from build123d import *

# Parameters (mm, degrees)
BOSS_EXTRUDE1_DEPTH = 6.35
SKETCH2_W           = 20
SKETCH2_H           = 6.55
CUT_EXTRUDE1_DEPTH  = 172.94569637
SKETCH4_W           = 6.55
SKETCH4_H           = 15
SKETCH4_W_2         = 6.35
CUT_EXTRUDE2_DEPTH  = 172.94569637
FILLET1_R           = 2


with BuildPart() as part:
    # Sketch1 → Boss-Extrude1 (new body)
    with BuildSketch(Plane(origin=(0, 0, 0), x_dir=(1, 0, 0), z_dir=(0, 1, 0))):
        Polygon((-170, 0), (-170, 20), (0, 20), (7, 20), (7, -25), (0, -25), (-170, -25), align=None)
    extrude(amount=BOSS_EXTRUDE1_DEPTH)

    # Sketch2 → Cut-Extrude1 (cut, through all)
    with BuildSketch(Plane(origin=(0, 6.35, 0), x_dir=(1, 0, 0), z_dir=(0, 1, 0))):
        with Locations((-110, -16.725)):
            Rectangle(SKETCH2_W, SKETCH2_H)
        with Locations((-155, -16.725)):
            Rectangle(SKETCH2_W, SKETCH2_H)
        with Locations((-65, -16.725)):
            Rectangle(SKETCH2_W, SKETCH2_H)
        with Locations((-20, -16.725)):
            Rectangle(SKETCH2_W, SKETCH2_H)
        with Locations((-110, -3.275)):
            Rectangle(SKETCH2_W, SKETCH2_H)
        with Locations((-155, -3.275)):
            Rectangle(SKETCH2_W, SKETCH2_H)
        with Locations((-65, -3.275)):
            Rectangle(SKETCH2_W, SKETCH2_H)
        with Locations((-20, -3.275)):
            Rectangle(SKETCH2_W, SKETCH2_H)
    extrude(amount=-CUT_EXTRUDE1_DEPTH, mode=Mode.SUBTRACT)

    # Sketch4 → Cut-Extrude2 (cut, through all)
    with BuildSketch(Plane(origin=(0, 6.35, 0), x_dir=(1, 0, 0), z_dir=(0, 1, 0))):
        with Locations((0, -12.5)):
            Rectangle(SKETCH4_W, SKETCH4_H)
        with Locations((0, 7.5)):
            Rectangle(SKETCH4_W_2, SKETCH4_H)
    extrude(amount=-CUT_EXTRUDE2_DEPTH, mode=Mode.SUBTRACT)

    # Fillet1
    fillet1_edges = [part.edges().sort_by_distance(p)[0] for p in [
        (7, 3.175, -20),
        (7, 3.175, 25),
        (-170, 3.175, 25),
        (-170, 3.175, -20),
    ]]
    fillet(fillet1_edges, radius=FILLET1_R)


solid = part.part
Could you check a few things on this model? Use its own coordinates, in mm. Coordinates: 2 decimals unless noted, no trailing zeros. Order: outer loops, then holes, each group sorted by start corner. A loop starts at its lowest first (then second) coordinate and runs counter-clockwise, first axis right, second up. Notation, with made-up numbers: (75.5, 16.25) -> (118.5, 16.25) arc R22 ccw to (118.5, 43.25) -> close; hole circle Ø10 at (87.25, 12.5). An arc over 180 degrees is marked (long way). One line per item, written item: value. Start each with the question number.
1) We'd pull the mould along X, two halves only. Please class faces 1 (the flat face through (0, 3, 0)), 2 (the flat face through (7, 3, 2)), 3 (the flat face through (-10, 3, 17)): +X half, -X half, draft (parallel to the pull), parting line (faces both ways), or undercut.
2) Imagine slicing it at A-A on x = -109. List the corners of the cut face in (y, z) for me, plus the area to 3 significant figures.
3) Imagine slicing it at C-C on y = 2. Count the separate pieces of the cut face and the enclosed holes in it, plus the area to 3 significant figures.
4) If I drill on L1, parallel to Z at x = -118, y = 2.5; L2, parallel to X at y = 5.25, z = 3.5; L3, parallel to X at y = 3, z = 16.5 (3 decimals), over which ranges is the centre line in solid material (lowest first)? Write a range as [from, to].
5) Imagine slicing it at B-B on z = -2. List the corners of the cut face in (x, y) for me (3 decimals), plus the area to 3 significant figures.
6) I'm going to push a flat-ended pin straight in: pin 1 (8 mm diameter, centred on x = -63, z = -8, fed in from -Y). Where does the tip first touch, or does it pass through?
Answer list:
1. face 1: undercut
1. face 2: +X half
1. face 3: undercut
2. outline: (0, -20) -> (6.35, -20) -> (6.35, 0) -> (0, 0) -> close; (0, 6.55) -> (6.35, 6.55) -> (6.35, 13.45) -> (0, 13.45) -> close; (0, 20) -> (6.35, 20) -> (6.35, 25) -> (0, 25) -> close
2. area: 203 mm2
3. separate pieces: 1
3. enclosed holes: 10
3. area: 6,720 mm2
4. L1: z = [-20, 0], [6.55, 13.45], [20, 25]
4. L2: x = [-170, -165], [-145, -120], [-100, -75], [-55, -30], [-10, 7]
4. L3: x = [-170, -165], [-145, -120], [-100, -75], [-55, -30], [-10, -3.275], [3.275, 7]
5. outline: (-170, 0) -> (-3.175, 0) -> (-3.175, 6.35) -> (-170, 6.35) -> close; (3.175, 0) -> (7, 0) -> (7, 6.35) -> (3.175, 6.35) -> close
5. area: 1,080 mm2
6. pin 1: stops at y = 0
